Read the model definition and answer for the solid it produces. Units are mm, in the model's axes. Coordinates: 2 decimals unless noted, no trailing zeros. Loops run counter-clockwise (first coordinate to the right, second up) from the corner with the lowest first, then second, coordinate; pieces in that order, holes last. Notation, with made-up numbers: (65.5, -18) - (122.5, -18) arc R21 cw to (122.5, -4) - close; hole circle Ø7 at (-25, 22). An arc over 180 degrees is marked (long way). Use one line per item in the form item = value.
from build123d import *

# Parameters (mm, degrees)
F0_W     = 18
F0_H     = 29.6524400212
F1_DEPTH = 9


# Not quite as in the source:
# - a feature names something its author has since deleted; it is built from what else it names


with BuildPart() as f1:
    # F0 (on Top) → F1 (new body)
    with BuildSketch(Plane.XY):
        with Locations((9, 14.8262200106)):
            Rectangle(F0_W, F0_H)
        with BuildLine():
            ThreePointArc((0, 29.6524400212), (-14.8262200106, 14.8262200106), (0, 0))
            Line((0, 0), (0, 29.6524400212))
        make_face()
        Polygon((18, 29.6524400212), (18, 0), (51, 0), (60, 8.7334750722), (60, 20.7334750722), (51, 29.6524400212), align=None)
    extrude(amount=F1_DEPTH)


solid = f1.part
Item 1: Find the intervals of material crossed by L1, parallel to X at y = 11.25, z = 5.75; L2, parallel to X at y = 18.75, z = 2.25; L3, parallel to Y at x = -2, z = 5.25, in increasing order.
Results below:
L1 = -14.39 to 60
L2 = -14.3 to 60
L3 = 0.14 to 29.52
Item 2: Each of these flat-tipped pins is pushed along its axis until it touches: P1, Ø2, axis at y = 7.5, z = 2, coming from the +X side; P2, Ø4, axis at y = 25, z = 3.5, coming from the -X side. Where does it stop, or does it pass through?
Results below:
P1 = 59.76
P2 = -12.37
Item 3: The part is cut by section B-B on y = 2.25. Give the vertices of the cut face in (x, z), plus the area to 3 significant figures.
Results below:
outline = (-7.85, 0) - (53.32, 0) - (53.32, 9) - (-7.85, 9) - close
area = 551 mm²
Item 4: For a pull along Z with two mould halves and no side action, classify faces 1 (the flat face through (22, 15, 9)), 2 (the flat face through (22, 15, 0)), 3 (the flat face through (26, 29.652, 4)) as +Z half, -Z half, draft (parallel to the pull), parting line (faces both ways), or undercut.
Results below:
face_1 = +Z half
face_2 = -Z half
face_3 = draft
Item 5: The part is cut by section C-C on y = 27.75. Give the vertices of the cut face in (x, z), plus the area to 3 significant figures.
Results below:
outline = (-7.27, 0) - (52.92, 0) - (52.92, 9) - (-7.27, 9) - close
area = 542 mm²
